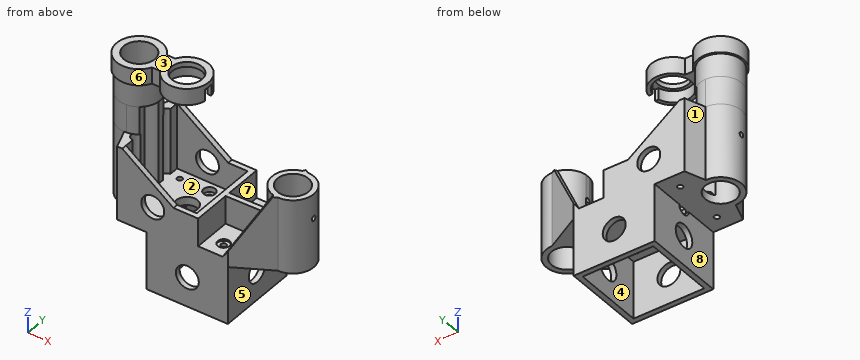
from build123d import *

# Parameters (mm, degrees)
SKETCH5_R       = 9.46
SKETCH5_R_2     = 1.6
EXTRUDE1_DEPTH  = 5
SKETCH6_R       = 9.46
EXTRUDE2_DEPTH  = 40
SKETCH7_W       = 49.45
SKETCH7_H       = 49.45
SKETCH7_W_2     = 43.1
SKETCH7_H_2     = 43.1
EXTRUDE3_DEPTH  = 35
EXTRUDE5_REACH  = 20.597
EXTRUDE6_REACH  = 20.597
SKETCH16_R      = 7
EXTRUDE9_DEPTH  = 49.45
EXTRUDE10_DEPTH = 17
SKETCH18_R      = 12.7
SKETCH18_R_2    = 9.46
EXTRUDE11_DEPTH = 14
SKETCH19_R      = 11.1
SKETCH19_R_2    = 9.46
EXTRUDE12_DEPTH = 7
SKETCH20_R      = 9.46
SKETCH20_R_2    = 9.2
EXTRUDE13_DEPTH = 3
EXTRUDE14_DEPTH = 15
SKETCH22_R      = 3.6
EXTRUDE15_DEPTH = 3
SKETCH23_R      = 3.6
EXTRUDE16_DEPTH = 3
SKETCH24_R      = 7
EXTRUDE17_DEPTH = 49.45
SKETCH25_R      = 6.5
EXTRUDE18_DEPTH = 5
EXTRUDE19_START = -25.300694
SKETCH26_R      = 1.5
EXTRUDE19_DEPTH = 119.050001
SKETCH27_R      = 3.6
EXTRUDE20_DEPTH = 1


with BuildPart() as part:
    # Sketch5 → Extrude1 (new body)
    with BuildSketch(Plane.XY):
        with BuildLine():
            Line((-21.825, -24.725), (0, -12.7))
            ThreePointArc((0, -12.7), (12.7, 0), (0, 12.7))
            Line((0, 12.7), (-21.825, 24.725))
            Line((-21.825, 24.725), (-89.375, 24.725))
            Line((-89.375, 24.725), (-93.65, 12.7))
            ThreePointArc((-93.65, 12.7), (-106.35, 0), (-93.65, -12.7))
            Line((-93.65, -12.7), (-89.375, -24.725))
            Line((-89.375, -24.725), (-21.825, -24.725))
        make_face()
        Circle(SKETCH5_R, mode=Mode.SUBTRACT)
        with Locations((-93.65, 0)):
            Circle(SKETCH5_R, mode=Mode.SUBTRACT)
        with Locations((-31.05, 15.5)):
            Circle(SKETCH5_R_2, mode=Mode.SUBTRACT)
        with Locations((-31.05, -15.5)):
            Circle(SKETCH5_R_2, mode=Mode.SUBTRACT)
        with Locations((-49.15, -15.5)):
            Circle(SKETCH5_R_2, mode=Mode.SUBTRACT)
        with Locations((-49.15, 15.5)):
            Circle(SKETCH5_R_2, mode=Mode.SUBTRACT)
        with Locations((-62.05, 15.5)):
            Circle(SKETCH5_R_2, mode=Mode.SUBTRACT)
        with Locations((-80.15, 15.5)):
            Circle(SKETCH5_R_2, mode=Mode.SUBTRACT)
        with Locations((-80.15, -15.5)):
            Circle(SKETCH5_R_2, mode=Mode.SUBTRACT)
        with Locations((-62.05, -15.5)):
            Circle(SKETCH5_R_2, mode=Mode.SUBTRACT)
    extrude(amount=EXTRUDE1_DEPTH)

    # Sketch6 → Extrude2 (add)
    with BuildSketch(Plane.XY.offset(5)):
        with BuildLine():
            Line((-39.925, 24.725), (-89.375, 24.725))
            Line((-89.375, 24.725), (-93.65, 12.7))
            ThreePointArc((-93.65, 12.7), (-106.35, 0), (-93.65, -12.7))
            Line((-93.65, -12.7), (-89.375, -24.725))
            Line((-89.375, -24.725), (-39.925, -24.725))
            Line((-39.925, -24.725), (-39.925, -1.585093616))
            Line((-39.925, -1.585093616), (-12.600693561, -1.585093616))
            ThreePointArc((-12.600693561, -1.585093616), (-9.51301391, -8.413831847), (-3.112651943, -12.312651943))
            Line((-3.112651943, -12.312651943), (-25, -24.725))
            Line((-25, -24.725), (-21.825, -24.725))
            Line((-21.825, -24.725), (0, -12.7))
            ThreePointArc((0, -12.7), (12.7, 0), (0, 12.7))
            Line((0, 12.7), (-21.825, 24.725))
            Line((-21.825, 24.725), (-25, 24.725))
            Line((-25, 24.725), (-3.112651943, 12.312651943))
            ThreePointArc((-3.112651943, 12.312651943), (-9.513885465, 8.41284633), (-12.601021697, 1.58248292))
            Line((-12.601021697, 1.58248292), (-39.925, 1.58248292))
            Line((-39.925, 1.58248292), (-39.925, 24.725))
        make_face()
        Circle(SKETCH6_R, mode=Mode.SUBTRACT)
        with BuildLine():
            Line((-86.2, -21.55), (-43.1, -21.55))
            Line((-43.1, -21.55), (-43.1, 21.55))
            Line((-43.1, 21.55), (-86.2, 21.55))
            Line((-86.2, 21.55), (-86.2, 15.891608363))
            ThreePointArc((-86.2, 15.891608363), (-89.375, 12.716608363), (-86.2, 9.541608363))
            Line((-86.2, 9.541608363), (-86.2, 5.830017153))
            ThreePointArc((-86.2, 5.830017153), (-103.11, 0), (-86.2, -5.830017153))
            Line((-86.2, -5.830017153), (-86.2, -9.508391637))
            ThreePointArc((-86.2, -9.508391637), (-89.375, -12.683391637), (-86.2, -15.858391637))
            Line((-86.2, -15.858391637), (-86.2, -21.55))
        make_face(mode=Mode.SUBTRACT)
    extrude(amount=EXTRUDE2_DEPTH)

    # Sketch7 → Extrude3 (add)
    with BuildSketch(Plane(origin=(0, 0, 0), x_dir=(-1, 0, 0), z_dir=(0, 0, -1))):
        with Locations((46.55, 0)):
            Rectangle(SKETCH7_W, SKETCH7_H)
        with Locations((46.55, 0)):
            Rectangle(SKETCH7_W_2, SKETCH7_H_2, mode=Mode.SUBTRACT)
    extrude(amount=EXTRUDE3_DEPTH)

    # Extrude5: up to this face of the body (flat: up to its plane)
    extrude5_end = Plane(part.part.faces().sort_by_distance((-10.9125, 18.7125, 22.5))[0])
    # Sketch12 → Extrude5 (cut, up to the picked face)
    with BuildSketch(Plane(origin=(4.5259255, 7.980803168, 0), x_dir=(0, 0, 1), z_dir=(-0.493298857, -0.869859895, 0)), mode=Mode.PRIVATE) as extrude5_sk1:
        Polygon((45, 8.781388226), (5, 33.943311626), (45, 33.943311626), align=None)
    extrude5_tool1 = split(extrude(extrude5_sk1.sketch, amount=-EXTRUDE5_REACH, mode=Mode.PRIVATE), bisect_by=extrude5_end, keep=Keep.BOTH, mode=Mode.PRIVATE)
    add(extrude5_tool1.solids().sort_by_distance((-17.704217, 20.587551, 31.666667))[0], mode=Mode.SUBTRACT)

    # Extrude6: up to this face of the body (flat: up to its plane)
    extrude6_end = Plane(part.part.faces().sort_by_distance((-10.9125, -18.7125, 22.5))[0])
    # Sketch13 → Extrude6 (cut, up to the picked face)
    with BuildSketch(Plane(origin=(4.5259255, -7.980803168, 0), x_dir=(0, 0, 1), z_dir=(-0.493298857, 0.869859895, 0)), mode=Mode.PRIVATE) as extrude6_sk1:
        Polygon((45, -8.781388226), (5, -33.943311626), (45, -33.943311626), align=None)
    extrude6_tool1 = split(extrude(extrude6_sk1.sketch, amount=-EXTRUDE6_REACH, mode=Mode.PRIVATE), bisect_by=extrude6_end, keep=Keep.BOTH, mode=Mode.PRIVATE)
    add(extrude6_tool1.solids().sort_by_distance((-17.704217, -20.587551, 31.666667))[0], mode=Mode.SUBTRACT)

    # Sketch16 → Extrude9 (cut)
    with BuildSketch(Plane.XZ.offset(24.725)):
        with Locations((-46.55, -17)):
            Circle(SKETCH16_R)
        with Locations((-67.618096531, 17)):
            Circle(SKETCH16_R)
        Polygon((-39.925, 22), (-16.781973348, 22.403360483), (-12.600693561, 29.053940018), (-12.600693561, 45), (-86.2, 45), (-54.981583076, 22), align=None)
    extrude(amount=-EXTRUDE9_DEPTH, mode=Mode.SUBTRACT)

    # Sketch17 → Extrude10 (add)
    with BuildSketch(Plane.XY.offset(45)):
        with BuildLine():
            Line((-86.2, 10.285305051), (-86.2, 5.830017153))
            ThreePointArc((-86.2, 5.830017153), (-103.11, 0), (-86.2, -5.830017153))
            Line((-86.2, -5.830017153), (-86.2, -10.285305051))
            ThreePointArc((-86.2, -10.285305051), (-89.146529591, -11.874710703), (-92.40601106, -12.638927625))
            ThreePointArc((-92.40601106, -12.638927625), (-106.334722718, -0.62274359), (-93.65, 12.7))
            ThreePointArc((-93.65, 12.7), (-89.734222565, 12.081253539), (-86.2, 10.285305051))
        make_face()
    extrude(amount=EXTRUDE10_DEPTH)

    # Sketch18 → Extrude11 (add)
    with BuildSketch(Plane.XY.offset(62)):
        with Locations((-93.65, 0)):
            Circle(SKETCH18_R)
        with Locations((-93.65, 0)):
            Circle(SKETCH18_R_2, mode=Mode.SUBTRACT)
    extrude(amount=EXTRUDE11_DEPTH)

    # Sketch19 → Extrude12 (add)
    with BuildSketch(Plane.XY.offset(76)):
        with BuildLine():
            Line((-81.398348387, -6.344577353), (-76.315821236, -6.344577353))
            ThreePointArc((-76.315821236, -6.344577353), (-51.370502761, 0), (-76.315821236, 6.344577353))
            Line((-76.315821236, 6.344577353), (-81.398348387, 6.344577353))
            ThreePointArc((-81.398348387, 6.344577353), (-107.446978982, 0), (-81.398348387, -6.344577353))
        make_face()
        with Locations((-64.65, 0)):
            Circle(SKETCH19_R, mode=Mode.SUBTRACT)
        with Locations((-93.65, 0)):
            Circle(SKETCH19_R_2, mode=Mode.SUBTRACT)
    extrude(amount=EXTRUDE12_DEPTH)

    # Sketch20 → Extrude13 (add)
    with BuildSketch(Plane.XY.offset(83)):
        with BuildLine():
            Line((-81.398348387, -6.344577353), (-76.315821236, -6.344577353))
            ThreePointArc((-76.315821236, -6.344577353), (-51.370502761, 0), (-76.315821236, 6.344577353))
            Line((-76.315821236, 6.344577353), (-81.398348387, 6.344577353))
            ThreePointArc((-81.398348387, 6.344577353), (-107.446978982, 0), (-81.398348387, -6.344577353))
        make_face()
        with Locations((-93.65, 0)):
            Circle(SKETCH20_R, mode=Mode.SUBTRACT)
        with Locations((-64.65, 0)):
            Circle(SKETCH20_R_2, mode=Mode.SUBTRACT)
    extrude(amount=EXTRUDE13_DEPTH)

    # Sketch21 → Extrude14 (cut)
    with BuildSketch(Plane.ZY.offset(43.1)):
        Polygon((76, 0), (76, -2.7), (83, -2.7), (83, 2.7), (76, 2.7), align=None)
    extrude(amount=EXTRUDE14_DEPTH, mode=Mode.SUBTRACT)

    # Sketch22 → Extrude15 (cut)
    with BuildSketch(Plane.XY.offset(5)):
        with Locations((-62.05, 15.5)):
            Circle(SKETCH22_R)
        with Locations((-62.05, -15.5)):
            Circle(SKETCH22_R)
    extrude(amount=-EXTRUDE15_DEPTH, mode=Mode.SUBTRACT)

    # Sketch23 → Extrude16 (cut)
    with BuildSketch(Plane(origin=(0, 0, 0), x_dir=(-1, 0, 0), z_dir=(0, 0, -1))):
        with Locations((49.15, 15.5)):
            Circle(SKETCH23_R)
        with Locations((49.15, -15.5)):
            Circle(SKETCH23_R)
    extrude(amount=-EXTRUDE16_DEPTH, mode=Mode.SUBTRACT)

    # Sketch24 → Extrude17 (cut)
    with BuildSketch(Plane.ZY.offset(71.275)):
        with Locations((-17, 0)):
            Circle(SKETCH24_R)
        with BuildLine():
            Line((0, 0), (0, 4))
            ThreePointArc((0, 4), (-4, 0), (0, -4))
            Line((0, -4), (0, 0))
        make_face()
    extrude(amount=-EXTRUDE17_DEPTH, mode=Mode.SUBTRACT)

    # Sketch25 → Extrude18 (cut)
    with BuildSketch(Plane(origin=(0, 0, 0), x_dir=(-1, 0, 0), z_dir=(0, 0, -1))):
        with Locations((46.55, 0)):
            Circle(SKETCH25_R)
        with Locations((64.65, 0)):
            Circle(SKETCH25_R)
    extrude(amount=-EXTRUDE18_DEPTH, mode=Mode.SUBTRACT)

    # Sketch26 → Extrude19 (cut)
    with BuildSketch(Plane.ZY.offset(12.600693561).offset(EXTRUDE19_START)):
        with Locations((30, 0)):
            Circle(SKETCH26_R)
    extrude(amount=EXTRUDE19_DEPTH, mode=Mode.SUBTRACT)

    # Sketch27 → Extrude20 (cut)
    with BuildSketch(Plane.XY.offset(5)):
        with Locations((-31.05, 15.5)):
            Circle(SKETCH27_R)
        with Locations((-31.05, -15.5)):
            Circle(SKETCH27_R)
    extrude(amount=-EXTRUDE20_DEPTH, mode=Mode.SUBTRACT)


solid = part.part
Input: part model. Units: mm. Frame: model coordinates. Face numbers are marked on the shaded views. A direction names the side the tool comes from. Round coordinates to 2 decimals unless told otherwise and drop trailing zeros. Order: outer loops, then holes, each group sorted by start corner. A loop starts at its lowest first (then second) coordinate and runs counter-clockwise, first axis right, second up.
1. Cut plane D-D, the plane x = -7. Output: boundary loops of the cut face in (y, z), then the cut area to 3 significant figures.
The answers:
outline: (-16.56, 0) - (-6.36, 0) - (-6.36, 45) - (-10.6, 45) - (-10.6, 5) - (-14.52, 5) - (-14.52, 37.9) - (-16.56, 36.3) - close; (6.36, 0) - (16.56, 0) - (16.56, 36.3) - (14.52, 37.9) - (14.52, 5) - (10.6, 5) - (10.6, 45) - (6.36, 45) - close
area: 572 mm2
2. Set-up query: the marked faces 4, 5, 6, 7 and 8. Return all of +Z, -Z, +X, -X, +Y, -Y with unobstructed straight access to the full face (end or side cutting, diameter ignored); none if empty.
The answers:
face 4: -Z
face 5: -Z, +X, +Y, -Y
face 6: +Z
face 7: +Z, +Y
face 8: -Z, -X, +Y, -Y
3. Pin query (flat end, axial travel): P1, Ø2.5, axis at x = -80, z = 79.5, coming from the +Y side; P2, Ø15, axis at x = -38, y = 6, coming from the -Z side; P3, Ø3, axis at y = -19, z = -18.5, coming from the +X side (3 decimals); P4, Ø3, axis at x = -49.15, y = -15.5, coming from the +Z side. Return the tip coordinate at first contact, or that it passes through.
The answers:
P1: stops at y = 6.34
P2: stops at z = 0
P3: stops at x = -21.825
P4: passes through
4. Cut plane A-A, the plane z = -17. Output: boundary loops of the cut face in (x, y) (3 decimals), then the cut area to 3 significant figures.
The answers:
outline: (-71.275, -24.725) - (-53.55, -24.725) - (-53.55, -21.55) - (-68.1, -21.55) - (-68.1, -7) - (-71.275, -7) - close; (-71.275, 7) - (-68.1, 7) - (-68.1, 21.55) - (-53.55, 21.55) - (-53.55, 24.725) - (-71.275, 24.725) - close; (-39.55, -24.725) - (-21.825, -24.725) - (-21.825, -7) - (-25, -7) - (-25, -21.55) - (-39.55, -21.55) - close; (-39.55, 21.55) - (-25, 21.55) - (-25, 7) - (-21.825, 7) - (-21.825, 24.725) - (-39.55, 24.725) - close
area: 410 mm2
5. Cut plane C-C, the plane z = 17. State how many separate pieces and enclosed holes the cut face has, then the cut area to 4 significant figures.
The answers:
separate pieces: 2
enclosed holes: 1
area: 992.5 mm2
6. Mould query, pull axis Z, two halves, no side actions, for the marked faces 1, 2 and 3. Classes: released by +Z, released by -Z, zero draft, split by the parting line, or undercut.
The answers:
face 1: zero draft
face 2: undercut
face 3: released by +Z
7. Material intervals for line 1 (X direction, y = 0.5, z = 64.5); line 2 (Z direction, x = -52.5, y = 3.5); line 3 (X direction, y = 16, z = 14) (3 decimals), sorted ascending.
The answers:
line 1: x = -106.34 to -103.1, -84.2 to -80.96
line 2: z = 0 to 5, 76 to 86
line 3: x = -92.477 to -86.2, -43.1 to -39.925, -9.615 to -5.989
8. Cut plane B-B, the plane x = 5.5. Output: boundary loops of the cut face in (y, z).
The answers:
outline: (-11.45, 0) - (-7.7, 0) - (-7.7, 45) - (-11.45, 45) - close; (7.7, 0) - (11.45, 0) - (11.45, 45) - (7.7, 45) - close
